Can you work these out from the model? Positions are in its coordinate system, mm. A direction names the side the tool comes from. Coordinates: 2 decimals unless noted, no trailing zeros. Loops run counter-clockwise (first coordinate to the right, second up) from the corner with the lowest first, then second, coordinate; pieces in that order, holes last. Notation, with made-up numbers: M 89,55.5 L 112,55.5 A25 ccw 112,89.5 Z; hole C 53.5,5.5 d10. An arc over 180 degrees is marked long. Return JSON: item names as keys, results as strings. Group by question number.
```python
from build123d import *

# Parameters (mm, degrees)
SKETCH1_R           = 10
BOSS_EXTRUDE1_DEPTH = 13
SKETCH2_R           = 2.5
CUT_EXTRUDE1_DEPTH  = 13
SKETCH3_R           = 4
CUT_EXTRUDE2_DEPTH  = 13


with BuildPart() as part:
    # Sketch1 → Boss-Extrude1 (new, symmetric)
    with BuildSketch(Plane(origin=(0, 0, 0), x_dir=(0, 0, -1), z_dir=(1, 0, 0))):
        with Locations(Location((0, 0, 0), (0, 0, 180))):
            Circle(SKETCH1_R)
    extrude(amount=BOSS_EXTRUDE1_DEPTH, both=True)

    # Sketch2 → Cut-Extrude1 (cut)
    with BuildSketch(Plane(origin=(13, 0, 0), x_dir=(0, 0, -1), z_dir=(1, 0, 0))):
        Circle(SKETCH2_R)
    extrude(amount=-CUT_EXTRUDE1_DEPTH, mode=Mode.SUBTRACT)

    # Sketch3 → Cut-Extrude2 (cut)
    with BuildSketch(Plane.ZY.offset(13)):
        Circle(SKETCH3_R)
    extrude(amount=-CUT_EXTRUDE2_DEPTH, mode=Mode.SUBTRACT)


solid = part.part
```
1) For faces 4 (the face through (6.59, -2.44, 0.54)), 5 (the face through (-6.591, -3.905, -0.867)), which set-ups out of +Z, -Z, +X, -X, +Y, -Y let a thin tool reach every point of the face, with its end or its side?
2) If I drill on line 1 (Y direction, x = -4, z = 0); line 2 (Y direction, x = 3.75, z = 0); line 3 (Z direction, x = 2, y = -1), over which ranges is the centre line in solid material (lowest first)? Write a range as from..to.
3) Suppose I cut it at C-C, the plane x = 8.5. List the corners of the cut face in (y, z) for me.
4) For pin 1 (1 mm diameter, centred on x = -2, y = -2.5, fed in from -Z); pin 2 (4 mm diameter, centred on x = -5, z = -6, fed in from -Y); pin 3 (12 mm diameter, centred on x = 1, y = 7.5, fed in from +Z), each with a flat end and sliding along its axis, tell me the tip position at first contact or that it passes through.
5) Suppose I cut it at A-A, the plane y = 0. List the corners of the cut face in (x, z) for me.
6) Suppose I cut it at D-D, the plane y = 3. List the corners of the cut face in (x, z) for me, then the cut area to 3 significant figures.
7) If we mould it in two halves opening along Z, with no side actions, what happens to faces 1 (the face through (0, 2, 2)), 2 (the face through (0, 0, -10)), 3 (the face through (13, 2, 2))? For each: +Z half, -Z half, draft (parallel to the pull), parting line (faces both ways), or undercut.
Returned:
{
 "1": {"face 4": "+X, -X", "face 5": "-X"},
 "2": {"line 1": "y = -10..-4, 4..10", "line 2": "y = -10..-2.5, 2.5..10", "line 3": "z = -9.95..-2.29, 2.29..9.95"},
 "3": {"outline": "C 0,0 d20; hole C 0,0 d5"},
 "4": {"pin 1": "stops at z = -9.8", "pin 2": "stops at y = -9.17", "pin 3": "stops at z = 9.89"},
 "5": {"outline": "M -13,-10 L 13,-10 L 13,-2.5 L 0,-2.5 L 0,-4 L -13,-4 Z; M -13,4 L 0,4 L 0,2.5 L 13,2.5 L 13,10 L -13,10 Z"},
 "6": {"outline": "M -13,-9.54 L 13,-9.54 L 13,9.54 L -13,9.54 L -13,2.65 L 0,2.65 L 0,-2.65 L -13,-2.65 Z", "area": "427 mm²"},
 "7": {"face 1": "undercut", "face 2": "parting line", "face 3": "draft"}
}
